Could you check a few things on this model? Use its own coordinates, in mm. Give positions to 0.01 mm unless a question says otherwise; leave off trailing zeros.
Autodesk Inventor part; units mm, degrees
ref_plane "YZ Plane" through (0, 0, 0) normal (1, 0, 0) x (0, 1, 0)
ref_plane "XZ Plane" through (0, 0, 0) normal (0, 1, 0) x (-1, 0, 0)
ref_plane "XY Plane" through (0, 0, 0) normal (0, 0, 1) x (1, 0, 0)
sketch "Sketch1" plane through (0, 0, 0) normal (0, 0, 1) x (1, 0, 0)
  line L0 (0, 0) -> (0, 15.0812)
  line L1 (0, 15.0812) -> (3.9624, 15.0812)
  line L2 (3.9624, 15.0812) -> (3.9624, 6.35)
  line L3 (3.9624, 6.35) -> (113.5126, 6.35)
  line L4 (113.5126, 6.35) -> (113.5126, 0)
  line L5 (113.5126, 0) -> (0, 0)
  line L6 (0, 17.4625) -> (113.5126, 17.4625)
  dimension "d0" = 15.0813
  dimension "d1" = 8.7312
  dimension "d2" = 6.35
  dimension "d3" = 113.5126
  dimension "d4" = 3.9624
  dimension "d5" = 113.5126
  dimension "d6" = 2.3813
revolve "Revolution1" add sketch "Sketch1" angle 360 about axis through (0, 17.4625, 0) along (1, 0, 0)
fillet "Fillet1" radius 6.35 1 edges at (0, 34.925, 0)
fillet "Fillet2" radius 6.35 1 edges at (113.5126, 34.925, 0)
properties part number "RubberHandleSleeveDE"
Item 1: We'd pull the mould along Y, two halves only. Please class faces 1 (the cylindrical face through (56.05, 34.91, 0.77)), 2 (the cylindrical face through (2.01, 19.84, -0.1)), 3 (the cylindrical face through (59.504, 25.653, -7.51)), 4 (the flat face through (0, 18, -3)): +Y half, -Y half, draft (parallel to the pull), parting line (faces both ways), or undercut.
Findings:
face 1: parting line
face 2: undercut
face 3: undercut
face 4: draft
Item 2: Please list where these lines run through material, in increasing order: line 1 along Z through (x, y) = (36, 17); line 2 along Y through (x, z) = (69, 0) (3 decimals); line 3 along X through (y, z) = (13, 6).
Findings:
line 1: z = -17.46 to -11.1, 11.1 to 17.46
line 2: y = 0 to 6.35, 28.575 to 34.925
line 3: x = 0 to 3.96
Item 3: For pin 1 (10 mm diameter, centred on x = 84.5, y = 24, fed in from -Z); pin 2 (20 mm diameter, centred on y = 17.46, z = 0, fed in from +X); pin 3 (4 mm diameter, centred on y = 7.5, z = -9, fed in from -X), each with a flat end and sliding along its axis, tell me the tip position at first contact or that it passes through.
Findings:
pin 1: stops at z = -17.39
pin 2: stops at x = 3.96
pin 3: stops at x = 0.01
